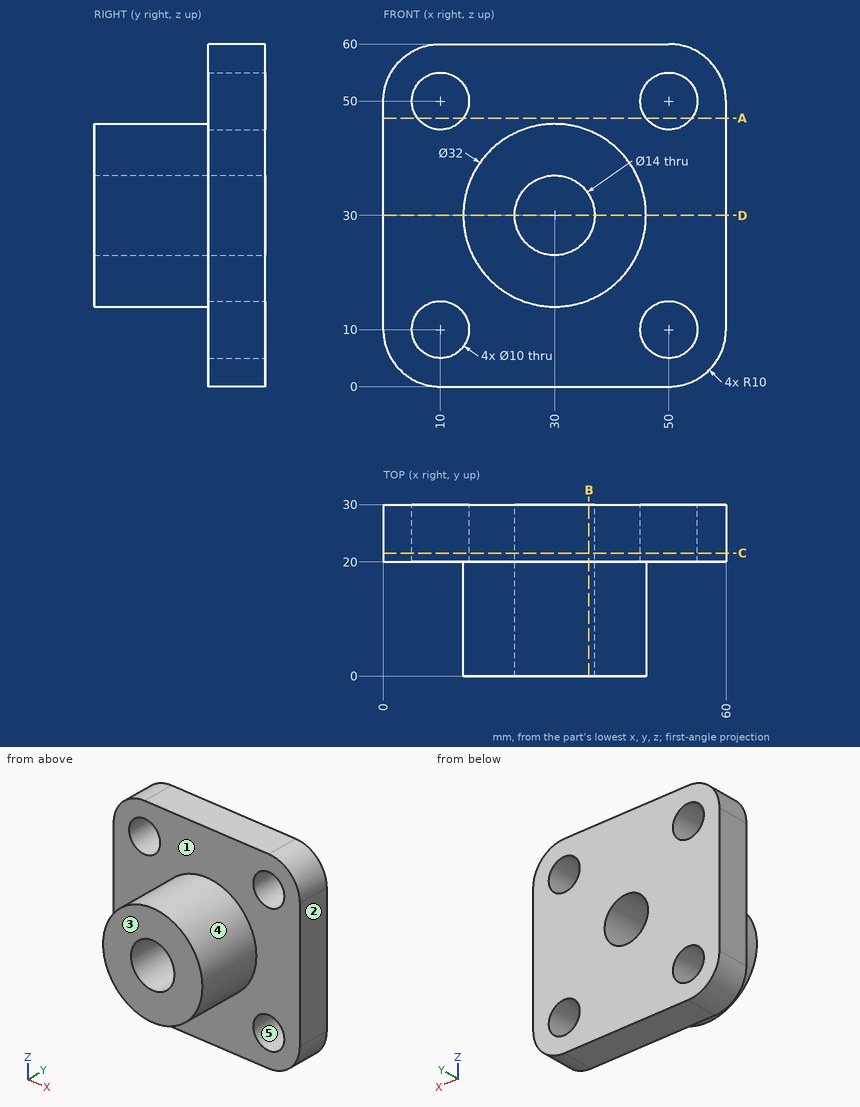
Here's the drawing with two shaded views (mm, measured from the low corner). I have some questions. A direction names the side the tool comes from. Round coordinates to 2 decimals unless told otherwise and drop trailing zeros. Loops run counter-clockwise (first coordinate to the right, second up) from the corner with the lowest first, then second, coordinate; pieces in that order, holes last.
1. If I drill on probe 1 along Z at (x, y) = (50, 26.5); probe 2 along X at (y, z) = (28.5, 51.5); probe 3 along Z at (x, y) = (48, 24.25), over which ranges is the centre line in solid material (lowest first)?
Answers:
probe 1: z = 0 to 5, 15 to 45, 55 to 60
probe 2: x = 0.11 to 5.23, 14.77 to 45.23, 54.77 to 59.89
probe 3: z = 0 to 5.42, 14.58 to 45.42, 54.58 to 60
2. Suppose I cut it at C-C, the plane y = 21.5. Please give me the cut outline in (x, z), and give its area (3 significant figures).
Answers:
outline: (0, 10) arc R10 ccw to (10, 0) - (50, 0) arc R10 ccw to (60, 10) - (60, 50) arc R10 ccw to (50, 60) - (10, 60) arc R10 ccw to (0, 50) - close; hole circle Ø10 at (10, 10); hole circle Ø10 at (10, 50); hole circle Ø14 at (30, 30); hole circle Ø10 at (50, 10); hole circle Ø10 at (50, 50)
area: 3,050 mm2
3. For the marked faces 1 and 2, which set-ups out of +Z, -Z, +X, -X, +Y, -Y let a thin tool reach every point of the face, with its end or its side?
Answers:
face 1: -Y
face 2: +Z, -Z, +X, +Y, -Y
4. Suppose I cut it at B-B, the plane x = 36. Please give me the cut outline in (y, z), and give its area (3 significant figures).
Answers:
outline: (0, 15.17) - (20, 15.17) - (20, 0) - (30, 0) - (30, 26.39) - (0, 26.39) - close; (0, 33.61) - (30, 33.61) - (30, 60) - (20, 60) - (20, 44.83) - (0, 44.83) - close
area: 977 mm2
5. Suppose I cut it at D-D, the plane z = 30. Please give me the cut outline in (x, y).
Answers:
outline: (0, 20) - (14, 20) - (14, 0) - (23, 0) - (23, 30) - (0, 30) - close; (37, 0) - (46, 0) - (46, 20) - (60, 20) - (60, 30) - (37, 30) - close
6. Will these pins go through, and if not, where does the flat tip stop? pin 1 (16 mm diameter, centred on x = 10, z = 10, fed in from -Y); pin 2 (2 mm diameter, centred on x = 7.5, z = 7, fed in from -Y); pin 3 (1 mm diameter, centred on y = 6.5, z = 24.5, fed in from +X); pin 4 (2 mm diameter, centred on y = 20, z = 52, fed in from -X).
Answers:
pin 1: stops at y = 20
pin 2: passes through
pin 3: stops at x = 45.2
pin 4: stops at x = 0.05
7. Suppose I cut it at A-A, the plane z = 47. Please give me the cut outline in (x, y), and give its area (3 significant figures).
Answers:
outline: (0, 20) - (6, 20) - (6, 30) - (0, 30) - close; (14, 20) - (46, 20) - (46, 30) - (14, 30) - close; (54, 20) - (60, 20) - (60, 30) - (54, 30) - close
area: 440 mm2
8. Thinking about a two-plate mould opening in X: for the marked faces 3, 4 and 5, which applies, released by +X, released by -X, zero draft, split by the parting line, or undercut?
Answers:
face 3: zero draft
face 4: split by the parting line
face 5: undercut
